from build123d import *

# Parameters (mm, degrees)
F1_DEPTH = 3.429


# Not quite as in the source:
# - ends of sketch curves that miss each other by under 0.0002 mm in the source are joined


with BuildPart() as f1:
    # F0 (on Front) → F1 (new body)
    with BuildSketch(Plane.XZ):
        with BuildLine():
            Line((412.522035, 410.7526964), (412.522035, 414.5626964))
            Line((412.522035, 414.5626964), (164.872035, 414.5626964))
            ThreePointArc((164.872035, 414.5626964), (139.472035, 389.1626964), (164.872035, 363.7626964))
            ThreePointArc((164.872035, 363.7626964), (184.4881935266, 369.6456603814), (197.6294252739, 385.352696025))
            Line((197.6294252739, 385.352696025), (164.872035, 385.3526964))
            Line((164.872035, 385.3526964), (164.872035, 389.1626964))
            Line((164.872035, 389.1626964), (412.522035, 389.1626964))
            Line((412.522035, 389.1626964), (412.522035, 392.9726964))
            Line((412.522035, 392.9726964), (418.872035, 392.9726964))
            Line((418.872035, 392.9726964), (418.872035, 410.7526964))
            Line((418.872035, 410.7526964), (412.522035, 410.7526964))
        make_face()
    extrude(amount=F1_DEPTH)


solid = f1.part
Source: CAD feature listing. Evaluate the final solid. Frame: model axes, mm. Give positions to 0.01 mm unless a question says otherwise; leave off trailing zeros. Write each loop counter-clockwise with the first axis right and the second up, starting at its lowest first coordinate (ties: lowest second). Pieces come first, ordered by that corner, then holes. Notation, with made-up numbers: M -29.75,-23.75 L 11.25,-23.75 A28 cw 11.25,1.25 Z; hole C -10.75,-29.5 d2. An arc over 180 degrees is marked long. Return JSON: item names as keys, results as strings. Group by question number.
1) Cut plane C-C, the plane z = 367.5. Output: boundary loops of the cut face in (x, y), plus the area to 4 significant figures.
2) Material intervals for line 1 along Z through (x, y) = (269.5, -0.3); line 2 along Z through (x, y) = (166.5, -2.7); line 3 along X through (y, z) = (-2.9, 389), sorted ascending. Write a range as [from, to].
3) Cut plane D-D, the plane z = 407. Output: boundary loops of the cut face in (x, y).
4) Pin query (flat end, axial travel): P1, Ø1.7, axis at x = 417, y = -2, coming from the -Z side; P2, Ø1, axis at y = -2, z = 391, coming from the +X side; P3, Ø2, axis at y = -1, z = 371.5, coming from the -X side; P4, Ø12, axis at x = 388.5, z = 377.5, coming from the -Y side. Return the tip coordinate at first contact, or that it passes through.
5) Cut plane B-B, the plane x = 195. Output: boundary loops of the cut face in (y, z).
6) Cut plane A-A, the plane y = -1.3. Output: boundary loops of the cut face in (x, z), plus the area to 3 significant figures.
Recorded:
{
 "1": {"outline": "M 151.61,-3.43 L 180.76,-3.43 L 180.76,0 L 151.61,0 Z", "area": "100.0 mm²"},
 "2": {"line 1": "z = [389.16, 414.56]", "line 2": "z = [363.8, 385.35], [389.16, 414.56]", "line 3": "x = [139.47, 164.87]"},
 "3": {"outline": "M 146.79,-3.43 L 418.87,-3.43 L 418.87,0 L 146.79,0 Z"},
 "4": {"P1": "stops at z = 392.97", "P2": "stops at x = 412.52", "P3": "stops at x = 145.7", "P4": "passes through"},
 "5": {"outline": "M -3.43,380.36 L 0,380.36 L 0,385.35 L -3.43,385.35 Z; M -3.43,389.16 L 0,389.16 L 0,414.56 L -3.43,414.56 Z"},
 "6": {"outline": "M 164.87,363.76 A35.65 ccw 197.63,385.35 L 164.87,385.35 L 164.87,389.16 L 412.52,389.16 L 412.52,392.97 L 418.87,392.97 L 418.87,410.75 L 412.52,410.75 L 412.52,414.56 L 164.87,414.56 A25.4 ccw Z", "area": "7,930 mm²"}
}
